Here's the drawing with two shaded views (mm, measured from the low corner). I have some questions. Coordinates: 2 decimals unless noted, no trailing zeros. Write each loop counter-clockwise with the first axis right and the second up, starting at its lowest first coordinate (ties: lowest second). Pieces come first, ordered by that corner, then holes. Notation, with made-up numbers: (78.25, 52) - (94.25, 52) arc R31 ccw to (94.25, 83) - close; hole circle Ø11 at (44.5, 60). An arc over 180 degrees is marked (long way). Answer in a Markdown table with one row per item. Add a question column.
Item 1: If I drill on probe 1 along Y at (x, z) = (115.5, 1.15); probe 2 along X at (y, z) = (72.5, 4); probe 3 along Y at (x, z) = (85.5, 2.65), over which ranges is the centre line in solid material (lowest first)? Write a range as from..to.
Item 2: I'm going to push flat-ended pins straight in: pin 1 (1.5 mm diameter, centred on x = 8, z = 2.5, fed in from +Y); pin 2 (1.5 mm diameter, centred on y = 152, z = 2, fed in from -X); pin 3 (1 mm diameter, centred on y = 55.5, z = 1.5, fed in from -X). Where does each tip first touch, or does it pass through?
Item 3: Imagine slicing it at B-B (z = 2.9). State how many separate pieces and enclosed holes the cut face has, plus the area to 3 significant figures.
Item 4: Imagine slicing it at A-A (y = 100.5). Please give me the cut outline in (x, z).
Item 5: Imagine slicing it at C-C (x = 97). Please give me the cut outline in (y, z).
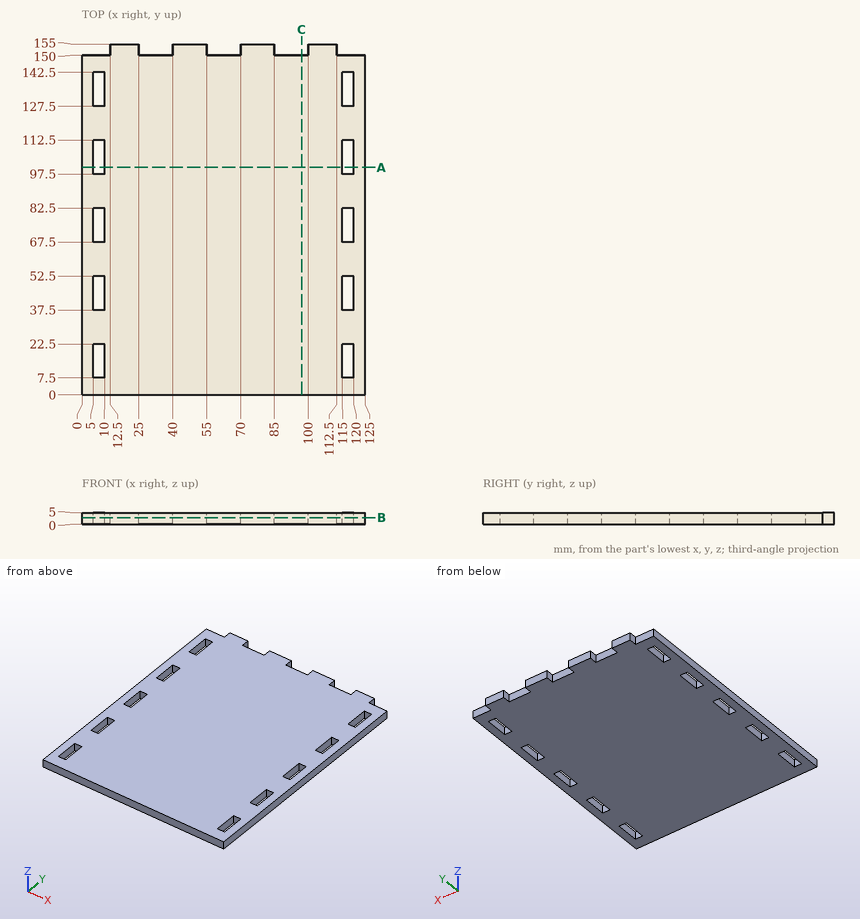
Here are the results:
| question | item | result |
|---|---|---|
| 1 | probe 1 | y = 0..7.5, 22.5..37.5, 52.5..67.5, 82.5..97.5, 112.5..127.5, 142.5..150 |
| 1 | probe 2 | x = 0..5, 10..115, 120..125 |
| 1 | probe 3 | y = 0..150 |
| 2 | pin 1 | stops at y = 150 |
| 2 | pin 2 | stops at x = 12.5 |
| 2 | pin 3 | stops at x = 0 |
| 3 | separate pieces | 1 |
| 3 | enclosed holes | 10 |
| 3 | area | 18,300 mm2 |
| 4 | outline | (0, 0) - (5, 0) - (5, 5) - (0, 5) - close; (10, 0) - (115, 0) - (115, 5) - (10, 5) - close; (120, 0) - (125, 0) - (125, 5) - (120, 5) - close |
| 5 | outline | (0, 0) - (150, 0) - (150, 5) - (0, 5) - close |
